from build123d import *

# Parameters (mm, degrees)
F0_R      = 2
F0_R_2    = 20
F1_DEPTH  = 4
F2_R      = 1.995
F3_DEPTH  = 4
F4_SIZE   = 1
F5_R      = 23.05
F5_R_2    = 20
F6_DEPTH  = 10
F8_DEPTH  = 2
F9_R      = 0.8
F10_DEPTH = 6


with BuildPart() as f1:
    # F0 (on Front) → F1 (new body)
    with BuildSketch(Plane.XZ):
        with BuildLine():
            ThreePointArc((29, 25), (27.828427, 27.828427), (25, 29))
            Line((25, 29), (-25, 29))
            ThreePointArc((-25, 29), (-27.828427, 27.828427), (-29, 25))
            Line((-29, 25), (-29, -25))
            ThreePointArc((-29, -25), (-27.828427, -27.828427), (-25, -29))
            Line((-25, -29), (25, -29))
            ThreePointArc((25, -29), (27.828427, -27.828427), (29, -25))
            Line((29, -25), (29, 25))
        make_face()
        with Locations((-25, -25)):
            Circle(F0_R, mode=Mode.SUBTRACT)
        with Locations((25, -25)):
            Circle(F0_R, mode=Mode.SUBTRACT)
        with Locations((-25, 25)):
            Circle(F0_R, mode=Mode.SUBTRACT)
        Circle(F0_R_2, mode=Mode.SUBTRACT)
        with Locations((25, 25)):
            Circle(F0_R, mode=Mode.SUBTRACT)
    extrude(amount=F1_DEPTH)

    # F2 (on face) → F3 (join)
    with BuildSketch(Plane(origin=(0, 0, 0), x_dir=(-1, 0, 0), z_dir=(0, 1, 0))):
        with Locations((-19, 25)):
            Circle(F2_R)
        with Locations((19, 25)):
            Circle(F2_R)
        with Locations((19, -25)):
            Circle(F2_R)
        with Locations((-16, -25)):
            Circle(F2_R)
    extrude(amount=F3_DEPTH)

    # F4
    f4_edges = [f1.edges().sort_by_distance(p)[0] for p in [
        (17.995, 4, -25),
        (-17.005, 4, -25),
        (-17.005, 4, 25),
        (20.995, 4, 25),
    ]]
    chamfer(f4_edges, length=F4_SIZE)

    # F5 (on face) → F6 (join)
    with BuildSketch(Plane.XZ.offset(4)):
        Circle(F5_R)
        Circle(F5_R_2, mode=Mode.SUBTRACT)
    extrude(amount=F6_DEPTH)

    # F7 (on face) → F8 (cut)
    with BuildSketch(Plane(origin=(0, 0, 0), x_dir=(-1, 0, 0), z_dir=(0, 1, 0))):
        with BuildLine():
            ThreePointArc((13, -15.198684), (0, -20), (-13, -15.198684))
            Line((-13, -15.198684), (-13, -23))
            ThreePointArc((-13, -23), (-12.414214, -24.414214), (-11, -25))
            Line((-11, -25), (11, -25))
            ThreePointArc((11, -25), (12.414214, -24.414214), (13, -23))
            Line((13, -23), (13, -15.198684))
        make_face()
    extrude(amount=-F8_DEPTH, mode=Mode.SUBTRACT)

    # F9 (on face) → F10 (cut)
    with BuildSketch(Plane(origin=(0, -2, 0), x_dir=(-1, 0, 0), z_dir=(0, 1, 0))):
        with Locations((-11.406512, -18.254235)):
            Circle(F9_R)
        with Locations((11.406512, -18.254235)):
            Circle(F9_R)
    extrude(amount=-F10_DEPTH, mode=Mode.SUBTRACT)


solid = f1.part
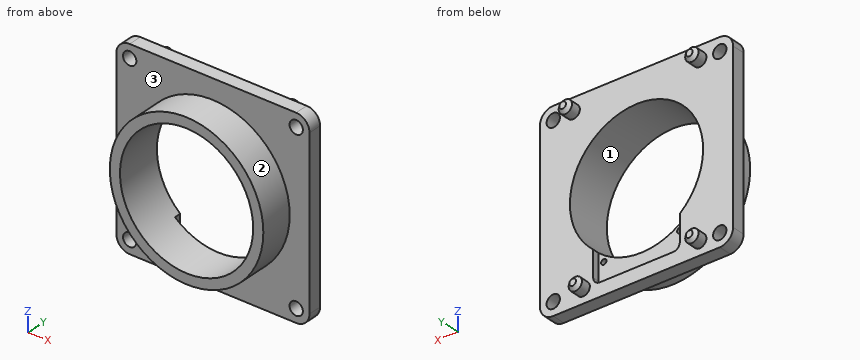
Build history of the part. All positions in model axes, mm. Face numbers are marked on the shaded views. Coordinates: 2 decimals unless noted, no trailing zeros. Order: outer loops, then holes, each group sorted by start corner. A loop starts at its lowest first (then second) coordinate and runs counter-clockwise, first axis right, second up. Notation, with made-up numbers: (78.5, -27) - (108.5, -27) arc R9 cw to (108.5, -22) - close; hole circle Ø4 at (11, -33.75). An arc over 180 degrees is marked (long way). Write item = value, one per line. Start each with the question number.
1) Two-plate mould, pull along Z, no slides. Class the marked faces 1, 2 and 3: pulls with the +Z half, pulls with the -Z half, needs draft (parallel to the pull), parting line crosses it, or undercut.
2) Saw through at D-D on y = -12. Write the cut outline in (x, z).
3) Saw through at B-B on y = -0.75. Write the cut outline in (x, z).
4) Flat gauge pins, fed straight in: pin 1 Ø4.5 at (x, z) = (-25, -25) entering from -Y; pin 2 Ø0.5 at (x, z) = (11.5, -18) entering from +Y; pin 3 Ø1 at (y, z) = (-9, 5.5) entering from -X. Where does each tip first touch, or does it go through?
5) Wall check: line 1 along Z through (x, y) = (25, -2.6); line 2 along Y through (x, z) = (26, -3.5); line 3 along Z through (x, y) = (0, -8). Give the ranges that are in metal, low to high. Write a range as from..to.
6) Saw through at C-C on z = -2. Write the cut outline in (x, y).
7) Saw through at A-A on x = 0. Write the cut outline in (y, z).
From the geometry:
q1.face_1 = undercut
q1.face_2 = parting line crosses it
q1.face_3 = needs draft
q2.outline = circle Ø46.1 at (0, 0); hole circle Ø40 at (0, 0)
q3.outline = (-29, -25) arc R4 ccw to (-25, -29) - (25, -29) arc R4 ccw to (29, -25) - (29, 25) arc R4 ccw to (25, 29) - (-25, 29) arc R4 ccw to (-29, 25) - close; hole circle Ø4 at (-25, -25); hole circle Ø4 at (-25, 25); hole (-13, -23) arc R2 ccw to (-11, -25) - (11, -25) arc R2 ccw to (13, -23) - (13, -15.2) arc R20 ccw (long way) to (-13, -15.2) - close; hole circle Ø4 at (25, -25); hole circle Ø4 at (25, 25)
q4.pin_1 = -4
q4.pin_2 = -8
q4.pin_3 = -22.5
q5.line_1 = -29..-27, -23..23, 27..29
q5.line_2 = -4..0
q5.line_3 = -23.05..-20, 20..23.05
q6.outline = (-29, -4) - (-22.96, -4) - (-22.96, -14) - (-19.9, -14) - (-19.9, 0) - (-29, 0) - close; (19.9, -14) - (22.96, -14) - (22.96, -4) - (29, -4) - (29, 0) - (19.9, 0) - close
q7.outline = (-14, -23.05) - (-4, -23.05) - (-4, -29) - (0, -29) - (0, -25) - (-2, -25) - (-2, -20) - (-14, -20) - close; (-14, 20) - (0, 20) - (0, 29) - (-4, 29) - (-4, 23.05) - (-14, 23.05) - close
